Read the model definition and answer for the solid it produces. Units are mm, in the model's axes. Coordinates: 2 decimals unless noted, no trailing zeros. Loops run counter-clockwise (first coordinate to the right, second up) from the corner with the lowest first, then second, coordinate; pieces in that order, holes last. Notation, with made-up numbers: (81, 29.5) -> (139, 29.5) arc R17 cw to (139, 43.5) -> close; hole circle Ø11 at (57, -17.75). An arc over 180 degrees is marked (long way). Answer as a JSON object with one key per item and string values. Group by question number.
1) Section C-C, the plane y = 0.3 is taken. Give the vertices of the cut face in (x, z) (3 decimals).
2) Section D-D, the plane z = -2.25 is taken. Give the vertices of the cut face in (x, y).
3) Consider probe 1 along Z at (x, y) = (0, 0.5); probe 2 along X at (y, z) = (0.55, -5.5); probe 3 along Z at (x, y) = (-10.25, 0.7). Determine where each line is inside the solid, lowest interval first. Write a range as [from, to].
4) Determine the mould class of faces 1 (the face through (-10.5, 0.49, -5.72)), 2 (the face through (-10.1, 0.5, 0)), 3 (the face through (0, 0, -8)) for opening direction Z: released by +Z, released by -Z, zero draft, split by the parting line, or undercut.
5) Section A-A, the plane z = -5.5 is taken. Give the vertices of the cut face in (x, y), plus the area to 3 significant figures.
6) Section B-B, the plane x = 0 is taken. Give the vertices of the cut face in (y, z).
from build123d import *

# Parameters (mm, degrees)
SKETCH1_R               = 12.7
BOSS_EXTRUDE1_DEPTH     = 1
CUT_EXTRUDE1_DEPTH      = 18.98832955
CUT_EXTRUDE1_DEPTH_BACK = 18.98832955
SKETCH19_R              = 1
CUT_EXTRUDE2_DEPTH      = 18.98832955
CUT_EXTRUDE2_DEPTH_BACK = 18.98832955
SKETCH20_R              = 7.5
SKETCH21_W              = 65.874202484
SKETCH21_H              = 51.979273979
CUT_EXTRUDE3_DEPTH      = 18.98832955
CUT_EXTRUDE4_DEPTH      = 18.98832955
CUT_EXTRUDE4_DEPTH_BACK = 18.98832955
SKETCH22_R              = 0.25


with BuildPart() as part:
    # Sketch1 → Boss-Extrude1 (new body)
    with BuildSketch(Plane(origin=(0, 0, 0), x_dir=(1, 0, 0), z_dir=(0, 1, 0))):
        with Locations(Location((0, 0, 0), (0, 0, 270))):
            Circle(SKETCH1_R)
    extrude(amount=BOSS_EXTRUDE1_DEPTH)

    # Sketch19 → Cut-Extrude1 (cut, two sides: drawn at the far end of the back side and taken through both)
    with BuildSketch(Plane(origin=(0, 1, 0), x_dir=(1, 0, 0), z_dir=(0, 1, 0)).offset(-CUT_EXTRUDE1_DEPTH_BACK)):
        with Locations(Location((0, 11, 0), (0, 0, 270))):
            Circle(SKETCH19_R)
        with Locations(Location((9.526279442, 5.5, 0), (0, 0, 270))):
            Circle(SKETCH19_R)
        with Locations(Location((9.526279442, -5.5, 0), (0, 0, 270))):
            Circle(SKETCH19_R)
        with Locations(Location((0, -11, 0), (0, 0, 270))):
            Circle(SKETCH19_R)
        with Locations(Location((-9.526279442, -5.5, 0), (0, 0, 270))):
            Circle(SKETCH19_R)
        with Locations(Location((-9.526279442, 5.5, 0), (0, 0, 270))):
            Circle(SKETCH19_R)
    extrude(amount=CUT_EXTRUDE1_DEPTH + CUT_EXTRUDE1_DEPTH_BACK, mode=Mode.SUBTRACT)

    # Sketch20 → Cut-Extrude2 (cut, two sides: drawn at the far end of the back side and taken through both)
    with BuildSketch(Plane(origin=(0, 1, 0), x_dir=(1, 0, 0), z_dir=(0, 1, 0)).offset(-CUT_EXTRUDE2_DEPTH_BACK)):
        with Locations(Location((0, 0, 0), (0, 0, 270))):
            Circle(SKETCH20_R)
    extrude(amount=CUT_EXTRUDE2_DEPTH + CUT_EXTRUDE2_DEPTH_BACK, mode=Mode.SUBTRACT)

    # Sketch21 → Cut-Extrude3 (cut, through all)
    with BuildSketch(Plane.XY):
        with Locations((-3.816154381, 6.321647006)):
            Rectangle(SKETCH21_W, SKETCH21_H)
    extrude(amount=CUT_EXTRUDE3_DEPTH, mode=Mode.SUBTRACT)

    # Sketch22 → Cut-Extrude4 (cut, two sides: drawn at the far end of the back side and taken through both)
    with BuildSketch(Plane(origin=(0, 1, 0), x_dir=(1, 0, 0), z_dir=(0, 1, 0)).offset(-CUT_EXTRUDE4_DEPTH_BACK)):
        with Locations(Location((-5.125, 8.876760389, 0), (0, 0, 270))):
            Circle(SKETCH22_R)
    extrude(amount=CUT_EXTRUDE4_DEPTH + CUT_EXTRUDE4_DEPTH_BACK, mode=Mode.SUBTRACT)


solid = part.part
Determined:
{
 "1": {"outline": "(-12.7, 0) arc R12.7 ccw to (12.7, 0) -> (7.5, 0) arc R7.5 cw to (-7.5, 0) -> close; hole circle Ø2 at (-9.526, -5.5); hole circle Ø0.5 at (-5.125, -8.877); hole circle Ø2 at (0, -11); hole circle Ø2 at (9.526, -5.5)"},
 "2": {"outline": "(-12.5, 0) -> (-7.15, 0) -> (-7.15, 1) -> (-12.5, 1) -> close; (7.15, 0) -> (12.5, 0) -> (12.5, 1) -> (7.15, 1) -> close"},
 "3": {"probe 1": "[-12.7, -12], [-10, -7.5]", "probe 2": "[-11.45, -10.53], [-8.53, -5.1], [5.1, 8.53], [10.53, 11.45]", "probe 3": "[-7.5, -6.19], [-4.81, 0]"},
 "4": {"face 1": "undercut", "face 2": "released by +Z", "face 3": "zero draft"},
 "5": {"outline": "(-11.45, 0) -> (-10.53, 0) -> (-10.53, 1) -> (-11.45, 1) -> close; (-8.53, 0) -> (-5.1, 0) -> (-5.1, 1) -> (-8.53, 1) -> close; (5.1, 0) -> (8.53, 0) -> (8.53, 1) -> (5.1, 1) -> close; (10.53, 0) -> (11.45, 0) -> (11.45, 1) -> (10.53, 1) -> close", "area": "8.70 mm²"},
 "6": {"outline": "(0, -12.7) -> (1, -12.7) -> (1, -12) -> (0, -12) -> close; (0, -10) -> (1, -10) -> (1, -7.5) -> (0, -7.5) -> close"}
}
